For this review, take the finished solid that the model builds, in its own axes (mm). Face numbers are marked on the shaded views. A direction names the side the tool comes from. Coordinates: 2 decimals unless noted, no trailing zeros. Loops run counter-clockwise (first coordinate to the right, second up) from the corner with the lowest first, then second, coordinate; pieces in that order, holes last. Notation, with made-up numbers: M -4,24 L 21,24 A33 ccw 21,53 Z; hole C 83.25,-3 d5. An arc over 180 degrees is marked long. Answer as a JSON object with one key per item and string values. Group by question number.
Item 1: Add section D-D (y = 4.5). State the section outline as (x, z) points.
Item 2: Insertion check: pin 1 (1.5 mm diameter, centred on x = -1, z = 24, fed in from -Y); pin 2 (4 mm diameter, centred on y = 14, z = -26, fed in from -X); pin 3 (7.5 mm diameter, centred on x = 1.5, y = 22.5, fed in from -Z). Each pin has a flat end and moves straight along its axis. Give the tip position at first contact, or say it passes through.
Item 3: Add section C-C (z = 5). State the section outline as (x, y) points, then the cut area to 3 significant figures.
Item 4: Add section A-A (y = -9). State the section outline as (x, z) points.
Item 5: Tool access review of the marked faces 1 and 2: name each direction out of +Z, -Z, +X, -X, +Y, -Y from which nothing blocks a thin tool from reaching the whole face with its end or side.
Item 6: Add section B-B (x = 23). State the section outline as (y, z) points, then the cut area to 3 significant figures.
Item 7: Wall thickness on L1, parallel to Y at x = -2, z = -18; L2, parallel to Y at x = 6.5, z = -8; L3, parallel to X at y = -11, z = 29.5: over which ranges is each line inside the solid? List them lowest first. Write a range as from..to.
Item 8: Mouldability with a two-part tool opening along Y and no side actions: class the marked faces 3, 4, 5 and 6 as +Y half, -Y half, draft (parallel to the pull), parting line (faces both ways), or undercut.
from build123d import *

# Parameters (mm, degrees)
SKETCH1_W           = 34
SKETCH1_H           = 6
BOSS_EXTRUDE2_DEPTH = 34
BOSS_EXTRUDE3_DEPTH = 34
CUT_EXTRUDE1_DEPTH  = 34
SKETCH10_W          = 9
SKETCH10_H          = 12
BOSS_EXTRUDE5_DEPTH = 34
CUT_EXTRUDE2_DEPTH  = 34


with BuildPart() as part:
    # Sketch1 → Boss-Extrude2 (new body)
    with BuildSketch(Plane.XY):
        with Locations((17, -3)):
            Rectangle(SKETCH1_W, SKETCH1_H)
    extrude(amount=BOSS_EXTRUDE2_DEPTH)

    # Sketch3 → Boss-Extrude3 (add)
    with BuildSketch(Plane.XY.offset(34)):
        Polygon((34, -6), (34, -15), (16, -15), (22, -6), align=None)
    extrude(amount=-BOSS_EXTRUDE3_DEPTH)

    # Sketch6 → section 0 of loft2
    with BuildSketch(Plane(origin=(0, 27, 0), x_dir=(1, 0, 0), z_dir=(0, 1, 0)), mode=Mode.PRIVATE) as loft2_s0:
        with BuildLine():
            Line((0, -9), (0, -24))
            Line((0, -24), (24, -24))
            Line((24, -24), (24, -9))
            Line((24, -9), (0, -9))
        make_face()
    # loft up to a face of the part (loft2)
    loft([loft2_s0.sketch, part.faces().sort_by_distance((17, 0, 17))[0]])

    # Sketch9 → Cut-Extrude1 (cut)
    with BuildSketch(Plane.ZY):
        Polygon((0, 0), (9, 0), (9, 27), align=None)
    extrude(amount=-CUT_EXTRUDE1_DEPTH, mode=Mode.SUBTRACT)

    # Sketch10 → Boss-Extrude5 (add)
    with BuildSketch(Plane.ZY):
        with Locations((4.5, 6)):
            Rectangle(SKETCH10_W, SKETCH10_H)
    extrude(amount=-BOSS_EXTRUDE5_DEPTH)

    # Sketch11 → Cut-Extrude2 (cut)
    with BuildSketch(Plane.XY.offset(9)):
        Polygon((34, 0), (34, 12), (29.555555556, 12), align=None)
    extrude(amount=-CUT_EXTRUDE2_DEPTH, mode=Mode.SUBTRACT)

    # Mirror1: part across plane


with BuildPart() as part_1:
    add(part.part)
    add(part.part.mirror(Plane(origin=(0, -6, 34), x_dir=(0, 0, 1), z_dir=(1, 0, 0))))

    # Mirror2: part across plane


with BuildPart() as part_2:
    add(part_1.part)
    add(part_1.part.mirror(Plane(origin=(0, 0, 0), x_dir=(1, 0, 0), z_dir=(0, 0, -1))))


solid = part_2.part
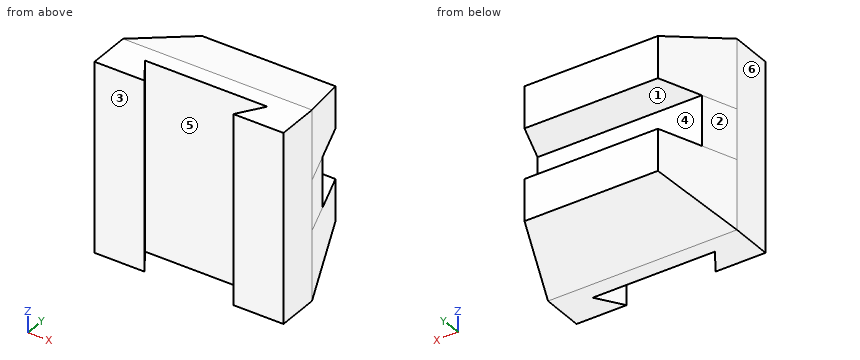
From the geometry:
{
 "1": {"outline": "M -32.33,-32.33 L 32.33,-32.33 L 32.33,32.33 L -32.33,32.33 Z"},
 "2": {"pin 1": "stops at y = -6", "pin 2": "stops at x = -29.56", "pin 3": "stops at z = -27.06"},
 "3": {"outline": "M -34,-15 L -16,-15 L -22,-6 L 22,-6 L 16,-15 L 34,-15 L 34,0 L 29.56,12 L -29.56,12 L -34,0 Z", "area": "1,440 mm²"},
 "4": {"outline": "M -34,-34 L -20,-34 L -20,34 L -34,34 Z; M 20,-34 L 34,-34 L 34,34 L 20,34 Z"},
 "5": {"face 1": "+X, -X, +Y", "face 2": "+Z, -Z, -X, +Y"},
 "6": {"outline": "M -15,-34 L 0,-34 L 27,-24 L 27,-9 L 12,-9 L 12,9 L 27,9 L 27,24 L 0,34 L -15,34 Z", "area": "2,320 mm²"},
 "7": {"L1": "y = -6..27", "L2": "y = -6..12", "L3": "x = -34..-18.67, 18.67..34"},
 "8": {"face 3": "-Y half", "face 4": "+Y half", "face 5": "undercut", "face 6": "draft"}
}
